CAD build for the part. Positions are in the model's coordinates, mm. A direction names the side the tool comes from. Give positions to 0.01 mm unless a question says otherwise; leave off trailing zeros. Order: outer loops, then holes, each group sorted by start corner. A loop starts at its lowest first (then second) coordinate and runs counter-clockwise, first axis right, second up. Notation, with made-up numbers: M 14.5,66.25 L 67.5,66.25 A12 ccw 67.5,82.25 Z; hole C -18.75,40.5 d9. An arc over 180 degrees is marked long. Put each result on its own line as item: value. Start each with the question number.
1) Cut at A-A (x = 0). Write the cut outline in (y, z).
2) Tool access for faces 4 (the face through (2, 0, 12)), 5 (the face through (-19.3, -19.2, -19.8)), 6 (the face through (-16, 16, -4.5)): list every direction of +Z, -Z, +X, -X, +Y, -Y with a clear straight run to the whole face (end or side of a thin tool).
3) Cut at C-C (z = 14). Write the cut outline in (x, y).
4) Cut at D-D (y = -7). Write the cut outline in (x, z), and give its area (3 significant figures).
5) Cut at B-B (y = -15.5). Write the cut outline in (x, z), and give its area (3 significant figures).
6) Two-plate mould, pull along X, no slides. Class faces 1 (the face through (16.15, -17.07, -2.28)), 2 (the face through (-21, 0, -19)), 3 (the face through (21, 0, -19)): released by +X, released by -X, zero draft, split by the parting line, or undercut.
7) Drill centre lines: line 1 (X direction, y = -15.5, z = -3.3); line 2 (X direction, y = 15, z = -2). Where is each one in solid material? Low to high. Write a range as [from, to].
8) Pin check, flat tips, straight feed: pin 1 (3.5 mm diameter, centred on x = -16.5, y = -16, fed in from +Z); pin 2 (3 mm diameter, centred on x = 15.5, y = 15.5, fed in from +Z); pin 3 (12 mm diameter, centred on y = 6, z = 6.5, fed in from +X). Stop position of each tip, or through.
Autodesk Inventor part; units mm, degrees
ref_plane "YZ Plane" through (0, 0, 0) normal (1, 0, 0) x (0, 1, 0)
ref_plane "XZ Plane" through (0, 0, 0) normal (0, 1, 0) x (-1, 0, 0)
ref_plane "XY Plane" through (0, 0, 0) normal (0, 0, 1) x (1, 0, 0)
sketch "Sketch1" plane through (0, 0, 0) normal (0, 0, 1) x (1, 0, 0)
  line L0 (21, -21) -> (-21, -21)
  line L1 (-21, -21) -> (-21, 21)
  line L2 (-21, 21) -> (21, 21)
  line L3 (21, 21) -> (21, -21)
  line L4 (21, -21) -> (-21, 21) construction
  line L5 (-21, -21) -> (21, 21) construction
  circle A0 centre (0, 0) radius 11
  circle A1 centre (0, 0) radius 2.5
  line L6 (2, 1.5) -> (2, -1.5)
  line L7 (0, 21) -> (0, -21) construction
  line L8 (-21, 0) -> (21, 0) construction
  point P0 (-15.5, 15.5)
  point P1 (15.5, 15.5)
  point P2 (15.5, -15.5)
  point P3 (-15.5, -15.5)
  dimension "d0" = 42
  dimension "d1" = 42
  dimension "d2" = 22
  dimension "d3" = 5
  dimension "d4" = 2
  dimension "d5" = 31
extrude "Extrusion1" add sketch "Sketch1" against normal blind 39 contours L0 L1 L2 L3 | A0 | A1 L6 | L6 A1
extrude "Extrusion2" add sketch "Sketch1" along normal blind 2 contours A0 | A1 L6 | L6 A1
extrude "Extrusion3" add sketch "Sketch1" along normal blind 22 contours L6 A1 picked at (0.2258, 0.7583)
hole "Hole1" at (-15.5, -15.5, 0) at (-15.5, 15.5, 0) at (15.5, 15.5, 0) at (15.5, -15.5, 0) direction (0, 0, -1) diameter 3.4 depth 4.5
chamfer "Chamfer1" distance 3.5 angle 45 4 edges at (-21, -21, -19.5) (-21, 21, -19.5) (21, -21, -19.5) (21, 21, -19.5)
properties part number "motor_x"
Solution:
1. outline: M -21,-39 L 21,-39 L 21,0 L 11,0 L 11,2 L 2.5,2 L 2.5,22 L -2.5,22 L -2.5,2 L -11,2 L -11,0 L -21,0 Z
2. face 4: +Z, +X, +Y, -Y
2. face 5: +Z, -Z, -X, -Y
2. face 6: +Z
3. outline: M 2,-1.5 L 2,1.5 A2.5 ccw long Z
4. outline: M -21,-39 L 21,-39 L 21,0 L 8.49,0 L 8.49,2 L -8.49,2 L -8.49,0 L -21,0 Z
4. area: 1,670 mm²
5. outline: M -21,-39 L 21,-39 L 21,0 L 17.2,0 L 17.2,-4.5 L 13.8,-4.5 L 13.8,0 L -13.8,0 L -13.8,-4.5 L -17.2,-4.5 L -17.2,0 L -21,0 Z
5. area: 1,610 mm²
6. face 1: undercut
6. face 2: released by -X
6. face 3: released by +X
7. line 1: [-21, -17.2], [-13.8, 13.8], [17.2, 21]
7. line 2: [-21, -17.12], [-13.88, 13.88], [17.12, 21]
8. pin 1: z = 0
8. pin 2: z = -4.5
8. pin 3: x = 10.81
